Part model, mm, in its own coordinate system. Face numbers are marked on the shaded views. Give positions to 0.01 mm unless a question says otherwise; leave off trailing zeros. Order: outer loops, then holes, each group sorted by start corner. A loop starts at its lowest first (then second) coordinate and runs counter-clockwise, first axis right, second up. Notation, with made-up numbers: (13.5, 40) -> (48.5, 40) arc R14 cw to (48.5, 52) -> close; hole circle Ø2 at (71.25, -20.5). An arc over 180 degrees is marked (long way). Write item = value, one per line. Start each with the question number.
Item 1: Drill centre lines: line 1 along Z through (x, y) = (24, -22); line 2 along X through (y, z) = (-6, 2.5); line 3 along Y through (x, z) = (-18.5, 6). Where is each one in solid material? Low to high.
Item 2: Pull direction Y, two halves, no side cores. Call the marked faces 1, 2 and 3: +Y half, -Y half, draft (parallel to the pull), parting line (faces both ways), or undercut.
Item 3: Flat gauge pins, fed straight in: P1, Ø4, axis at x = -11, y = -2, coming from the +Z side; P2, Ø1.5, axis at y = -0.5, z = 5.5, coming from the +X side; P3, Ø1, axis at x = -2.5, z = 6.5, coming from the -Y side. Where does each tip first touch, or does it go through?
Item 4: Band-saw the part on C-C on z = 4.25. Write the cut outline in (x, y) (3 decimals).
Item 5: Band-saw the part on B-B on x = -2.5. Write the cut outline in (y, z).
Item 6: Band-saw the part on A-A on y = -11.5. Write the cut outline in (x, z), plus the area to 3 significant figures.
```python
from build123d import *

# Parameters (mm, degrees)
F1_DEPTH     = 7.4836481363
F2_R         = 5.08
F3_T1_DEPTH  = 47.6248391628
F3_T3_DEPTH  = 112.7664723158
F3_T6_ANGLE  = 90
F3_T8_ANGLE  = 90
F3_T10_ANGLE = 90
F3_T12_ANGLE = 90
F4_W         = 62.8648391628
F4_H         = 91.2811607122
F5_DEPTH     = 0.7581766695


# Not quite as in the source:
# - a fillet or chamfer that OpenCascade refuses, or shapes differently, is made with other operations: its cross-section is extruded or revolved along the edge and cut away or added


with BuildPart() as f1:
    # F0 (on Top) → F1 (new body)
    with BuildSketch(Plane.XY):
        with BuildLine():
            ThreePointArc((36.5124195814, 56.3832361579), (32.7926757025, 65.363492279), (23.8124195814, 69.0832361579))
            Line((23.8124195814, 69.0832361579), (-23.8124195814, 69.0832361579))
            ThreePointArc((-23.8124195814, 69.0832361579), (-32.7926757025, 65.363492279), (-36.5124195814, 56.3832361579))
            Line((-36.5124195814, 56.3832361579), (-36.5124195814, -56.3832361579))
            ThreePointArc((-36.5124195814, -56.3832361579), (-32.7926757025, -65.363492279), (-23.8124195814, -69.0832361579))
            Line((-23.8124195814, -69.0832361579), (23.8124195814, -69.0832361579))
            ThreePointArc((23.8124195814, -69.0832361579), (32.7926757025, -65.363492279), (36.5124195814, -56.3832361579))
            Line((36.5124195814, -56.3832361579), (36.5124195814, 56.3832361579))
        make_face()
    extrude(amount=F1_DEPTH)

    # F2
    f2_edges = [f1.edges().sort_by_distance(p)[0] for p in [
        (0, -69.083236, 7.483648),
    ]]
    fillet(f2_edges, radius=F2_R)

    # F3: fillet of radius 5.08 on 1 edges, made by hand

    # F3_s2 → F3_t1 (cut)
    with BuildSketch(Plane.YZ.offset(-23.8124195814)):
        with BuildLine():
            ThreePointArc((-64.7654194988, 0), (-67.2363032003, 0.6414040808), (-69.0832361579, 2.4036481363))
            Line((-69.0832361579, 2.4036481363), (-69.0832361579, 0))
            Line((-69.0832361579, 0), (-64.7654194988, 0))
        make_face()
        with BuildLine():
            ThreePointArc((64.7654194988, 0), (67.2363032003, 0.6414040808), (69.0832361579, 2.4036481363))
            Line((69.0832361579, 2.4036481363), (69.0832361579, 0))
            Line((69.0832361579, 0), (64.7654194988, 0))
        make_face()
    extrude(amount=F3_T1_DEPTH, mode=Mode.SUBTRACT)

    # F3_s4 → F3_t3 (cut)
    with BuildSketch(Plane.XZ.offset(-56.3832361579)):
        with BuildLine():
            ThreePointArc((36.5124195814, 2.4036481363), (34.6654866238, 0.6414040808), (32.1946029223, 0))
            Line((32.1946029223, 0), (36.5124195814, 0))
            Line((36.5124195814, 0), (36.5124195814, 2.4036481363))
        make_face()
        with BuildLine():
            ThreePointArc((-32.1946029223, 0), (-34.6654866238, 0.6414040808), (-36.5124195814, 2.4036481363))
            Line((-36.5124195814, 2.4036481363), (-36.5124195814, 0))
            Line((-36.5124195814, 0), (-32.1946029223, 0))
        make_face()
    extrude(amount=F3_T3_DEPTH, mode=Mode.SUBTRACT)

    # F3_s5 → F3_t6 (revolve, cut)
    with BuildSketch(Plane.XZ.offset(56.3832361579)):
        with BuildLine():
            ThreePointArc((-32.1946029223, 0), (-34.6654866238, 0.6414040808), (-36.5124195814, 2.4036481363))
            Line((-36.5124195814, 2.4036481363), (-36.5124195814, 0))
            Line((-36.5124195814, 0), (-32.1946029223, 0))
        make_face()
    revolve(axis=Axis((-23.8124195814, -56.3832361579, 0), (0, 0, 1)), revolution_arc=F3_T6_ANGLE, mode=Mode.SUBTRACT)

    # F3_s7 → F3_t8 (revolve, cut)
    with BuildSketch(Plane.YZ.offset(23.8124195814)):
        with BuildLine():
            ThreePointArc((-64.7654194988, 0), (-67.2363032003, 0.6414040808), (-69.0832361579, 2.4036481363))
            Line((-69.0832361579, 2.4036481363), (-69.0832361579, 0))
            Line((-69.0832361579, 0), (-64.7654194988, 0))
        make_face()
    revolve(axis=Axis((23.8124195814, -56.3832361579, 0), (0, 0, 1)), revolution_arc=F3_T8_ANGLE, mode=Mode.SUBTRACT)

    # F3_s9 → F3_t10 (revolve, cut)
    with BuildSketch(Plane.XZ.offset(-56.3832361579)):
        with BuildLine():
            ThreePointArc((36.5124195814, 2.4036481363), (34.6654866238, 0.6414040808), (32.1946029223, 0))
            Line((32.1946029223, 0), (36.5124195814, 0))
            Line((36.5124195814, 0), (36.5124195814, 2.4036481363))
        make_face()
    revolve(axis=Axis((23.8124195814, 56.3832361579, 0), (0, 0, 1)), revolution_arc=F3_T10_ANGLE, mode=Mode.SUBTRACT)

    # F3_s11 → F3_t12 (revolve, cut)
    with BuildSketch(Plane.YZ.offset(-23.8124195814)):
        with BuildLine():
            ThreePointArc((64.7654194988, 0), (67.2363032003, 0.6414040808), (69.0832361579, 2.4036481363))
            Line((69.0832361579, 2.4036481363), (69.0832361579, 0))
            Line((69.0832361579, 0), (64.7654194988, 0))
        make_face()
    revolve(axis=Axis((-23.8124195814, 56.3832361579, 0), (0, 0, 1)), revolution_arc=F3_T12_ANGLE, mode=Mode.SUBTRACT)

    # F4 (on face) → F5 (cut)
    with BuildSketch(Plane.XY.offset(7.4836481363)):
        Rectangle(F4_W, F4_H)
    extrude(amount=-F5_DEPTH, mode=Mode.SUBTRACT)


solid = f1.part
```
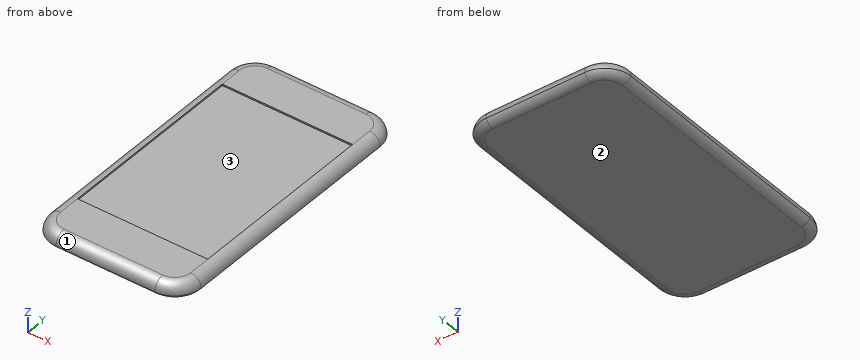
Values found:
q1.line_1 = 0 to 6.73
q1.line_2 = -36.51 to 36.51
q1.line_3 = -67.59 to 67.59
q2.face_1 = -Y half
q2.face_2 = draft
q2.face_3 = undercut
q3.P1 = 6.73
q3.P2 = 35.94
q3.P3 = -67.59
q4.outline = (-36.165, -56.383) arc R12.353 ccw to (-23.812, -68.736) -> (23.812, -68.736) arc R12.353 ccw to (36.165, -56.383) -> (36.165, 56.383) arc R12.353 ccw to (23.812, 68.736) -> (-23.812, 68.736) arc R12.353 ccw to (-36.165, 56.383) -> close
q5.outline = (-69.08, 2.4) arc R5.08 ccw to (-64.77, 0) -> (64.77, 0) arc R5.08 ccw to (69.08, 2.4) arc R5.08 ccw to (64, 7.48) -> (45.64, 7.48) -> (45.64, 6.73) -> (-45.64, 6.73) -> (-45.64, 7.48) -> (-64, 7.48) arc R5.08 ccw to start
q6.outline = (-36.51, 2.4) arc R5.08 ccw to (-32.19, 0) -> (32.19, 0) arc R5.08 ccw to (36.51, 2.4) arc R5.08 ccw to (31.43, 7.48) -> (31.43, 6.73) -> (-31.43, 6.73) -> (-31.43, 7.48) arc R5.08 ccw to start
q6.area = 482 mm^2
